from build123d import *

# Parameters (mm, degrees)
SKETCH1_W           = 300
SKETCH1_H           = 600
BOSS_EXTRUDE1_DEPTH = 50
SKETCH2_W           = 300
SKETCH2_H           = 500
CUT_EXTRUDE1_DEPTH  = 30
SKETCH3_W           = 50
SKETCH3_H           = 500
BOSS_EXTRUDE2_DEPTH = 36
FILLET1_R           = 20


with BuildPart() as part:
    # Sketch1 → Boss-Extrude1 (new body)
    with BuildSketch(Plane(origin=(0, 0, 0), x_dir=(1, 0, 0), z_dir=(0, 1, 0))):
        with Locations((29.676258993, 266.816546763)):
            Rectangle(SKETCH1_W, SKETCH1_H)
    extrude(amount=BOSS_EXTRUDE1_DEPTH)

    # Sketch2 → Cut-Extrude1 (cut)
    with BuildSketch(Plane(origin=(0, 0, 0), x_dir=(-1, 0, 0), z_dir=(0, -1, 0))):
        with Locations((-29.676258993, 266.816546763)):
            Rectangle(SKETCH2_W, SKETCH2_H)
    extrude(amount=-CUT_EXTRUDE1_DEPTH, mode=Mode.SUBTRACT)

    # Sketch3 → Boss-Extrude2 (add)
    with BuildSketch(Plane(origin=(0, 0, 0), x_dir=(-1, 0, 0), z_dir=(0, -1, 0))):
        with Locations((-29.676258993, 266.816546763)):
            Rectangle(SKETCH3_W, SKETCH3_H)
    extrude(amount=-BOSS_EXTRUDE2_DEPTH)

    # Fillet1
    fillet1_edges = [part.edges().sort_by_distance(p)[0] for p in [
        (-120.323741007, 0, 8.183453237),
        (179.676258993, 0, -541.816546763),
        (-57.823741007, 0, -516.816546763),
        (117.176258993, 0, -16.816546763),
        (117.176258993, 0, -516.816546763),
        (-57.823741007, 0, -16.816546763),
        (4.676258993, 0, -266.816546763),
        (54.676258993, 0, -266.816546763),
        (29.676258993, 0, -566.816546763),
        (179.676258993, 0, 8.183453237),
        (29.676258993, 0, 33.183453237),
        (-120.323741007, 0, -541.816546763),
    ]]
    fillet(fillet1_edges, radius=FILLET1_R)


solid = part.part
Input: part model. Units: mm. Frame: model coordinates. A direction names the side the tool comes from. Coordinates: 2 decimals unless noted, no trailing zeros. Order: outer loops, then holes, each group sorted by start corner. A loop starts at its lowest first (then second) coordinate and runs counter-clockwise, first axis right, second up.
1. Draft query along Z for faces 4 (the flat face through (28, 35, -566.817)), 5 (the cylindrical face through (10.69, 5.703, -270.597)), 6 (the flat face through (-57, 30, -270)), 7 (the cylindrical face through (175.932, 8.349, 7.833)). Return one class per face: +Z half, -Z half, draft (parallel to the pull), parting line (faces both ways), or undercut.
Checked values:
face 4: -Z half
face 5: undercut
face 6: undercut
face 7: draft
2. Cut plane C-C, the plane y = 10. Return loops of the section in (x, z), plus the area to 3 significant figures.
Checked values:
outline: (-117.64, -564.14) - (177, -564.14) - (177, -519.5) - (52, -519.5) - (52, -14.14) - (177, -14.14) - (177, 30.5) - (-117.64, 30.5) - (-117.64, -14.14) - (7.36, -14.14) - (7.36, -519.5) - (-117.64, -519.5) - close
area: 48,900 mm2
3. Cut plane A-A, the plane x = 117. Return loops of the section in (y, z), plus the area to 3 significant figures.
Checked values:
outline: (0, -546.82) arc R20 ccw to (20, -566.82) - (50, -566.82) - (50, 33.18) - (20, 33.18) arc R20 ccw to (0, 13.18) - (0, 3.18) arc R20 ccw to (20, -16.82) - (30, -16.82) - (30, -516.82) - (20, -516.82) arc R20 ccw to (0, -536.82) - close
area: 14,700 mm2
4. Contact query for flat-ended pins moving along their axis: P1, Ø12, axis at x = 8, y = 17.5, coming from the -Z side; P2, Ø5, axis at x = -10, z = -320, coming from the -Y side; P3, Ø11, axis at y = 22.5, z = -238.5, coming from the +X side; P4, Ø5, axis at y = 23, z = -182.5, coming from the -X side. Output: stop coordinate, or through.
Checked values:
P1: stops at z = -566.82
P2: stops at y = 30
P3: stops at x = 54.68
P4: stops at x = 4.68
5. Cut plane B-B, the plane z = -211. Return loops of the section in (x, y), plus the area to 3 significant figures.
Checked values:
outline: (-120.32, 30) - (4.68, 30) - (4.68, 20) arc R20 ccw to (24.68, 0) - (34.68, 0) arc R20 ccw to (54.68, 20) - (54.68, 30) - (179.68, 30) - (179.68, 50) - (-120.32, 50) - close
area: 7,330 mm2
6. Access query for faces 1 (the flat face through (118, 30, -270)), 2 (the flat face through (30, 0, -393)), 3 (the cylindrical face through (-48.8, 5.7, -10.8)). Directions: +Z, -Z, +X, -X, +Y, -Y. A direction counts if a zero-diameter tool reaches every point of the face in a straight line with its end or side. Return the directions, or none.
Checked values:
face 1: +X, -Y
face 2: +Z, -Z, +X, -X, -Y
face 3: -X, -Y
7. Ray query, line 1 along Z through (x, y) = (133, 27); line 2 along Z through (x, y) = (-66.5, 18); line 3 along Y through (x, z) = (-100.5, -459). Return the intervals inside material, ascending.
Checked values:
line 1: z = -566.82 to -516.82, -16.82 to 33.18
line 2: z = -566.72 to -516.92, -16.72 to 33.08
line 3: y = 30 to 50
